The figure shows three views and two pictorial views of one solid part (mm, origin at its lowest corner). Answer the questions. A direction names the side the tool comes from. Coordinates: 2 decimals unless noted, no trailing zeros. Order: outer loops, then holes, each group sorted by start corner. A loop starts at its lowest first (then second) coordinate and runs counter-clockwise, first axis right, second up. Notation, with made-up numbers: (7.25, 30.25) -> (41.25, 30.25) arc R19 cw to (41.25, 44.25) -> close; hole circle Ø2 at (60.5, 58.5). An arc over 180 degrees is marked (long way). Write item = value, one per line. Start each with the question number.
Q1. Which of the six approach directions +Z, -Z, +X, -X, +Y, -Y give full straight-line access (tool end or side, diameter ignored) to the marked faces 1, 2 and 3?
Q2. The part is cut by section C-C, the plane x = 45. Determine the outline of the cut face in (y, z), plus the area to 3 significant figures.
Q3. Straight lines are drawn through the part: L1, parallel to X at y = 15.25, z = 16 (1 decimal); L2, parallel to Z at x = 10, y = 14; L3, parallel to Z at x = 11, y = 16.75. For each, find the intervals that lie inside material, in ascending order. Write a range as from..to.
Q4. Flat-ended cylindrical pins translate along their axes: pin 1 (3 mm diameter, centred on x = 11.5, y = 11.5, fed in from +Z) (1 decimal); pin 2 (5.5 mm diameter, centred on y = 6.5, z = 33, fed in from +X) (3 decimals); pin 3 (10.5 mm diameter, centred on x = 3.5, y = 13.5, fed in from -Z). Find the tip coordinate at first contact, or state that the pin passes through.
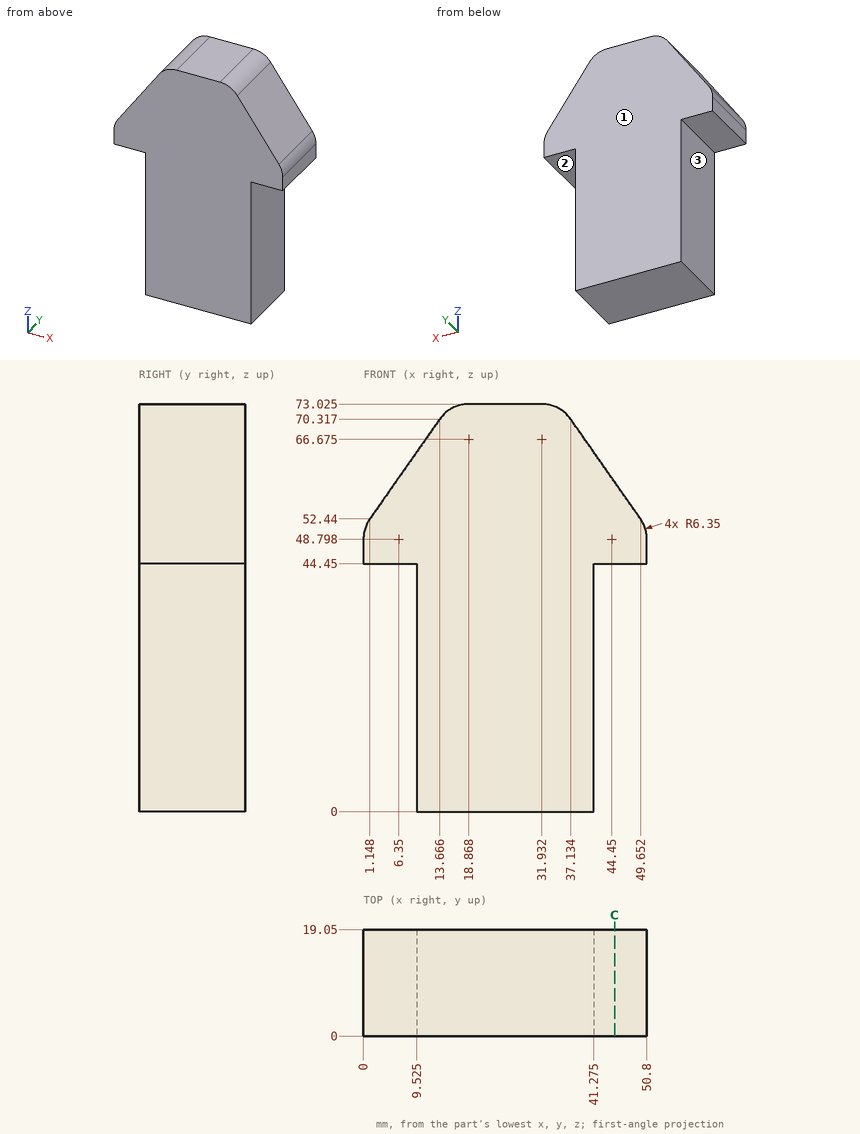
Model answer:
q1.face_1 = +Z, -Z, +X, -X, +Y
q1.face_2 = -Z, +X, +Y, -Y
q1.face_3 = -Z, -X, +Y, -Y
q2.outline = (0, 44.45) -> (19.05, 44.45) -> (19.05, 59.08) -> (0, 59.08) -> close
q2.area = 279 mm2
q3.L1 = 9.5..41.3
q3.L2 = 0..65.08
q3.L3 = 0..66.51
q4.pin_1 = 69.4
q4.pin_2 = 41.275
q4.pin_3 = 44.45
